from build123d import *

# Parameters (mm, degrees)
CUT_EXTRUDE1_DEPTH = 1.5


with BuildPart() as part:
    # Sketch2 → Revolve1 (revolve)
    with BuildSketch(Plane(origin=(0, 0, 0), x_dir=(0, 0, -1), z_dir=(1, 0, 0)), mode=Mode.PRIVATE) as revolve1_sk:
        with BuildLine():
            Line((-16.25, 0), (-16.25, 2.125))
            Line((-16.25, 2.125), (-16.125, 2.25))
            Line((-16.125, 2.25), (-13.875, 2.25))
            Line((-13.875, 2.25), (-13.75, 2.125))
            Line((-13.75, 2.125), (-13.75, 1.375))
            ThreePointArc((-13.75, 1.375), (-13.713388348, 1.286611652), (-13.625, 1.25))
            Line((-13.625, 1.25), (15.957716426, 1.25))
            Line((15.957716426, 1.25), (16.25, 0.957716426))
            Line((16.25, 0.957716426), (16.25, 0))
            Line((16.25, 0), (-16.25, 0))
        make_face()
    revolve(revolve1_sk.sketch.rotate(Axis((0, 0, -16.25), (0, 0, 1)), 90), axis=Axis((0, 0, -16.25), (0, 0, 1)))

    # Sketch3 → Cut-Extrude1 (cut)
    with BuildSketch(Plane.XY.offset(16.25)):
        Polygon((1, -0.577350269), (1, 0.577350269), (0, 1.154700538), (-1, 0.577350269), (-1, -0.577350269), (0, -1.154700538), align=None)
    extrude(amount=-CUT_EXTRUDE1_DEPTH, mode=Mode.SUBTRACT)

    # Cut-Extrude2 cone 1 section (through the dimple's axis) → Cut-Extrude2 (revolve, cut)
    with BuildSketch(Plane(origin=(0, 0, 16.25), x_dir=(0, -1, 0), z_dir=(1, 0, 0))):
        Polygon((0, 0), (1.241303079, 0), (0, 1.241303079), align=None)
    revolve(axis=Axis((0, 0, 16.25), (0, 0, -1)), mode=Mode.SUBTRACT)


solid = part.part
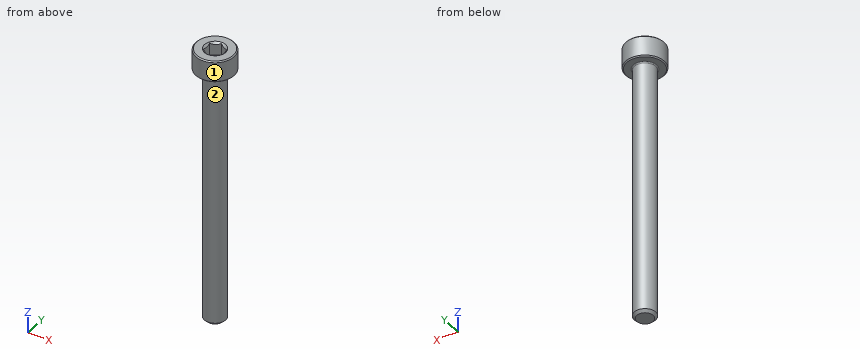
Could you check a few things on this model? Use its own coordinates, in mm. Face numbers are marked on the shaded views. A direction names the side the tool comes from. Give positions to 0.01 mm unless a question says otherwise; leave off trailing zeros. Order: outer loops, then holes, each group sorted by start corner. A loop starts at its lowest first (then second) coordinate and runs counter-clockwise, first axis right, second up.
1. I need wall thicknesses on L1, parallel to Z at x = -0.85, y = -0.45; L2, parallel to Z at x = -1.9, y = -0.65; L3, parallel to X at y = 0.8, z = 11.5. Which ranges of each line are inside material? Lowest first, please.
Answers below:
L1: z = -16.25 to 14.75
L2: z = 13.75 to 16.25
L3: x = -0.96 to 0.96
2. For pin 1 (2 mm diameter, centred on y = 1.5, z = -6, fed in from -X); pin 2 (0.6 mm diameter, centred on x = 0, y = 0, fed in from +Z); pin 3 (1 mm diameter, centred on y = -1, z = -1, fed in from +X), each with a flat end and sliding along its axis, tell me the tip position at first contact or that it passes through.
Answers below:
pin 1: stops at x = -1.15
pin 2: stops at z = 14.75
pin 3: stops at x = 1.15
3. Suppose I cut it at B-B (z = -9). Write out the boundary of the cut face in (x, y), plus the area to 3 significant figures.
Answers below:
outline: circle Ø2.5 at (0, 0)
area: 4.91 mm2
4. Suppose I cut it at A-A (y = 0). Write out the boundary of the cut face in (x, z) (3 decimals).
Answers below:
outline: (-2.25, 13.875) - (-2.125, 13.75) - (-1.375, 13.75) arc R0.125 cw to (-1.25, 13.625) - (-1.25, -15.958) - (-0.958, -16.25) - (0.958, -16.25) - (1.25, -15.958) - (1.25, 13.625) arc R0.125 cw to (1.375, 13.75) - (2.125, 13.75) - (2.25, 13.875) - (2.25, 16.125) - (2.125, 16.25) - (1.241, 16.25) - (1, 16.009) - (1, 14.75) - (-1, 14.75) - (-1, 16.009) - (-1.241, 16.25) - (-2.125, 16.25) - (-2.25, 16.125) - close
5. Which directions (+Z, -Z, +X, -X, +Y, -Y) give clear straight access to the entire face, cutting with the end or side of a thin tool? Please do the marked faces 1 and 2.
Answers below:
face 1: +Z, -Z
face 2: -Z
